```python
from build123d import *

# Parameters (mm, degrees)
F0_W      = 140.6558603048
F0_H      = 61.1045844853
F1_DEPTH  = 30
F2_R      = 19
F3_W      = 102.6558603048
F3_H      = 23.1045844853
F4_DEPTH  = 25
F5_W      = 4.1960617527
F5_H      = 7.4001618195
F6_DEPTH  = 55.3
F7_W      = 69.3877674639
F7_H      = 13.8425575569
F8_DEPTH  = 54.5
F9_R      = 3.055172352
F10_DEPTH = 61.9
F11_W     = 6.6588682532
F11_H     = 3.1128286794
F11_H_2   = 3.8515164927
F11_W_2   = 6.1259952784
F11_H_3   = 4.1949943118
F11_H_4   = 5.4464771822
F12_DEPTH = 20
F13_R     = 1.4165828047
F14_DEPTH = 15


with BuildPart() as f1:
    # F0 (on Front) → F1 (new body)
    with BuildSketch(Plane.XZ):
        Rectangle(F0_W, F0_H)
    extrude(amount=F1_DEPTH)

    # F2
    f2_edges = [f1.edges().sort_by_distance(p)[0] for p in [
        (0, -30, 30.552292),
        (-70.32793, -30, 0),
        (0, -30, -30.552292),
        (70.32793, -30, 0),
    ]]
    fillet(f2_edges, radius=F2_R)

    # F3 (on face) → F4 (cut)
    with BuildSketch(Plane.XZ.offset(30)):
        Rectangle(F3_W, F3_H)
    extrude(amount=-F4_DEPTH, mode=Mode.SUBTRACT)

    # F5 (on face) → F6 (cut)
    with BuildSketch(Plane(origin=(51.3279301524, 0, 0), x_dir=(0, -1, 0), z_dir=(-1, 0, 0))):
        with Locations((9.8722497933, 0.9650638094)):
            Rectangle(F5_W, F5_H)
    extrude(amount=-F6_DEPTH, mode=Mode.SUBTRACT)

    # F7 (on face) → F8 (cut)
    with BuildSketch(Plane(origin=(0, 0, 11.5522922426), x_dir=(1, 0, 0), z_dir=(0, 0, -1))):
        with Locations((0.842327252, 16.1106861196)):
            Rectangle(F7_W, F7_H)
    extrude(amount=-F8_DEPTH, mode=Mode.SUBTRACT)

    # F9 (on face) → F10 (cut)
    with BuildSketch(Plane(origin=(0, 0, 11.5522922426), x_dir=(1, 0, 0), z_dir=(0, 0, -1))):
        with Locations((-46.420622617, 25.4190824926)):
            Circle(F9_R)
    extrude(amount=-F10_DEPTH, mode=Mode.SUBTRACT)

    # F11 (on face) → F12 (join)
    with BuildSketch(Plane.XZ.offset(5)):
        with Locations((-47.9984960258, -9.995877903)):
            Rectangle(F11_W, F11_H)
        with Locations((-47.9984960258, 9.6265339963)):
            Rectangle(F11_W, F11_H_2)
        with Locations((48.2649325132, 9.4547950868)):
            Rectangle(F11_W_2, F11_H_3)
        with Locations((48.2649325132, -8.8290536515)):
            Rectangle(F11_W_2, F11_H_4)
    extrude(amount=F12_DEPTH)

    # F13 (on face) → F14 (cut)
    with BuildSketch(Plane.XZ.offset(25)):
        with Locations((-47.9030236602, 9.6265339963)):
            Circle(F13_R)
    extrude(amount=-F14_DEPTH, mode=Mode.SUBTRACT)


solid = f1.part
```
Part model, mm, in its own coordinate system. A direction names the side the tool comes from. Give positions to 0.01 mm unless a question says otherwise; leave off trailing zeros. Loops run counter-clockwise (first coordinate to the right, second up) from the corner with the lowest first, then second, coordinate; pieces in that order, holes last. Notation, with made-up numbers: M 35,89.5 L 47,89.5 A20 ccw 47,101.5 Z; hole C -33,13 d8. An arc over 180 degrees is marked long. Return JSON: item names as keys, results as strings.
1) 3-axis set-ups, long thin cutter, end or side, ignore diameter. For faces 4 (the face through (35.536, -16, 21)), 5 (the face through (-44.669, -15, -10)), 6 (the face through (0.985, -26.443, 22.621)), 7 (the face through (61, -11.97, 1)): which of +Z, -Z, +X, -X, +Y, -Y reach the whole face in a straight line?
Calculated:
{"face 4": "+Z", "face 5": "-Y", "face 6": "+Z, +X, -X, -Y", "face 7": "+X"}
2) Pull direction X, two halves, no side cores. Call faces 1 (the face through (51.328, -20, 0)), 2 (the face through (-70.328, -5, 0)), 3 (the face through (-1, -5, 30.552)): released by +X, released by -X, zero draft, split by the parting line, or undercut.
Calculated:
{"face 1": "undercut", "face 2": "released by -X", "face 3": "zero draft"}
3) Saw through at B-B, the plane x = -11.5. List the corners of the cut face in (y, z), then the cut area to 3 significant figures.
Calculated:
{"outline": "M -30,-11.55 A19 ccw -11,-30.55 L 0,-30.55 L 0,30.55 L -9.19,30.55 L -9.19,11.55 L -5,11.55 L -5,-11.55 Z; M -30,11.55 L -23.03,11.55 L -23.03,26.26 A19 ccw Z", "area": "854 mm2"}
4) Saw through at A-A, the plane z = 1. List the corners of the cut face in (x, y), then the cut area to 3 significant figures.
Calculated:
{"outline": "M -70.33,-11 A19 ccw -51.33,-30 L -51.33,-5 L 51.33,-5 L 51.33,-7.77 L 70.33,-7.77 L 70.33,0 L -70.33,0 Z; M 51.33,-30 A19 ccw 70.3,-11.97 L 51.33,-11.97 Z", "area": "1,420 mm2"}
5) Drill centre lines: line 1 (Z direction, x = 33.5, y = -7); line 2 (X direction, y = -10, z = -6); line 3 (Y direction, x = 0, z = -9). Where is each one in solid material? Low to high.
Calculated:
{"line 1": "z = -30.55 to -11.55, 11.55 to 30.55", "line 2": "x = -70.33 to -51.33, 51.33 to 70.33", "line 3": "y = -5 to 0"}
6) Flat gauge pins, fed straight in: pin 1 Ø8 at (y, z) = (-23, -23.5) entering from +X; pin 2 Ø2 at (x, z) = (59, 0.5) entering from -Y; pin 3 Ø5 at (x, y) = (49, -17.5) entering from -Z; pin 4 Ø6 at (x, z) = (45.5, -2) entering from +Y. Where does each tip first touch, or does it go through?
Calculated:
{"pin 1": "stops at x = 68.56", "pin 2": "stops at y = -28.79", "pin 3": "stops at z = -30.13", "pin 4": "stops at y = 0"}
7) Saw through at D-D, the plane z = 20.5. List the corners of the cut face in (x, y).
Calculated:
{"outline": "M -70.33,-11 A19 ccw -60.28,-27.76 L -48.38,-27.76 A3.06 cw long -44.46,-27.76 L 60.28,-27.76 A19 ccw 70.33,-11 L 70.33,0 L -70.33,0 Z; hole M -33.85,-23.03 L 35.54,-23.03 L 35.54,-9.19 L -33.85,-9.19 Z"}
8) Saw through at C-C, the plane y = -6.5. List the corners of the cut face in (x, z).
Calculated:
{"outline": "M -70.33,-30.55 L 70.33,-30.55 L 70.33,30.55 L -70.33,30.55 Z; hole M -51.33,-8.44 L -44.67,-8.44 L -44.67,-11.55 L 45.2,-11.55 L 45.2,-6.11 L 51.33,-6.11 L 51.33,7.36 L 45.2,7.36 L 45.2,11.55 L -44.67,11.55 L -44.67,7.7 L -51.33,7.7 Z"}
